```python
from build123d import *

# Parameters (mm, degrees)
F0_W     = 1004.8875
F0_H     = 609.6
F0_W_2   = 184.15
F0_H_2   = 95.25
F0_W_3   = 171.45
F0_H_3   = 88.9
F0_W_4   = 230.1875
F0_H_4   = 114.3
F0_H_5   = 60.325
F0_H_6   = 92.075
F1_DEPTH = 76.2
F2_W     = 1004.8875
F2_H     = 609.6
F3_DEPTH = 12.7
F5_DEPTH = 12.7


with BuildPart() as f1:
    # F0 (on Top) → F1 (new body)
    with BuildSketch(Plane.XY):
        with Locations((-595.931344, -92.764258)):
            Rectangle(F0_W, F0_H)
        with Locations((-993.600094, -337.239258)):
            Rectangle(F0_W_2, F0_H_2, mode=Mode.SUBTRACT)
        with Locations((-799.925094, -337.239258)):
            Rectangle(F0_W_2, F0_H_2, mode=Mode.SUBTRACT)
        with Locations((-612.600094, -340.414258)):
            Rectangle(F0_W_3, F0_H_3, mode=Mode.SUBTRACT)
        with Locations((-993.600094, -232.464258)):
            Rectangle(F0_W_2, F0_H_2, mode=Mode.SUBTRACT)
        with Locations((-993.600094, -127.689258)):
            Rectangle(F0_W_2, F0_H_2, mode=Mode.SUBTRACT)
        with Locations((-799.925094, -232.464258)):
            Rectangle(F0_W_2, F0_H_2, mode=Mode.SUBTRACT)
        with Locations((-612.600094, -241.989258)):
            Rectangle(F0_W_3, F0_H_3, mode=Mode.SUBTRACT)
        with Locations((-799.925094, -127.689258)):
            Rectangle(F0_W_2, F0_H_2, mode=Mode.SUBTRACT)
        with Locations((-612.600094, -143.564258)):
            Rectangle(F0_W_3, F0_H_3, mode=Mode.SUBTRACT)
        with Locations((-431.625094, -340.414258)):
            Rectangle(F0_W_3, F0_H_3, mode=Mode.SUBTRACT)
        with Locations((-221.281344, -327.714258)):
            Rectangle(F0_W_4, F0_H_4, mode=Mode.SUBTRACT)
        with Locations((-431.625094, -241.989258)):
            Rectangle(F0_W_3, F0_H_3, mode=Mode.SUBTRACT)
        with Locations((-431.625094, -143.564258)):
            Rectangle(F0_W_3, F0_H_3, mode=Mode.SUBTRACT)
        with Locations((-221.281344, -203.889258)):
            Rectangle(F0_W_4, F0_H_4, mode=Mode.SUBTRACT)
        with Locations((-993.600094, -22.914258)):
            Rectangle(F0_W_2, F0_H_2, mode=Mode.SUBTRACT)
        with Locations((-799.925094, -22.914258)):
            Rectangle(F0_W_2, F0_H_2, mode=Mode.SUBTRACT)
        with Locations((-612.600094, -45.139258)):
            Rectangle(F0_W_3, F0_H_3, mode=Mode.SUBTRACT)
        with Locations((-612.600094, 53.285742)):
            Rectangle(F0_W_3, F0_H_3, mode=Mode.SUBTRACT)
        with Locations((-993.600094, 81.860742)):
            Rectangle(F0_W_2, F0_H_2, mode=Mode.SUBTRACT)
        with Locations((-993.600094, 169.173242)):
            Rectangle(F0_W_2, F0_H_5, mode=Mode.SUBTRACT)
        with Locations((-799.925094, 81.860742)):
            Rectangle(F0_W_2, F0_H_2, mode=Mode.SUBTRACT)
        with Locations((-799.925094, 169.173242)):
            Rectangle(F0_W_2, F0_H_5, mode=Mode.SUBTRACT)
        with Locations((-612.600094, 153.298242)):
            Rectangle(F0_W_3, F0_H_6, mode=Mode.SUBTRACT)
        with Locations((-431.625094, -45.139258)):
            Rectangle(F0_W_3, F0_H_3, mode=Mode.SUBTRACT)
        with Locations((-431.625094, 53.285742)):
            Rectangle(F0_W_3, F0_H_3, mode=Mode.SUBTRACT)
        with Locations((-221.281344, -80.064258)):
            Rectangle(F0_W_4, F0_H_4, mode=Mode.SUBTRACT)
        with Locations((-221.281344, 43.760742)):
            Rectangle(F0_W_4, F0_H_4, mode=Mode.SUBTRACT)
        with Locations((-431.625094, 153.298242)):
            Rectangle(F0_W_3, F0_H_6, mode=Mode.SUBTRACT)
        with Locations((-221.281344, 154.885742)):
            Rectangle(F0_W_4, F0_H_3, mode=Mode.SUBTRACT)
    extrude(amount=F1_DEPTH)

    # F2 (on face) → F3 (join)
    with BuildSketch(Plane(origin=(0, 0, 0), x_dir=(1, 0, 0), z_dir=(0, 0, -1))):
        with Locations((-595.931344, 92.764258)):
            Rectangle(F2_W, F2_H)
    extrude(amount=F3_DEPTH)

    # F4 (on face) → F5 (join)
    with BuildSketch(Plane(origin=(0, 0, -12.7), x_dir=(1, 0, 0), z_dir=(0, 0, -1))):
        Polygon((-1098.375094, 397.564258), (-1098.375094, -212.035742), (-1085.675094, -212.035742), (-1085.675094, 384.864258), (-106.187594, 384.864258), (-106.187594, -212.035742), (-93.487594, -212.035742), (-93.487594, 397.564258), align=None)
    extrude(amount=F5_DEPTH)


solid = f1.part
```
Check sheet for the modelled part. Datum: model origin and axes. Units: mm. Give positions to 0.01 mm unless a question says otherwise; leave off trailing zeros. Write each loop counter-clockwise with the first axis right and the second up, starting at its lowest first coordinate (ties: lowest second). Pieces come first, ordered by that corner, then holes.
Item 1: Gauge pin test, flat ends, axial feed: pin 1 (6 mm diameter, centred on x = -897.5, y = -24.5, fed in from -Z); pin 2 (5 mm diameter, centred on x = -199, y = 24.5, fed in from +Z). Record the tip position at first contact, or that the pin passes through.
Item 2: Draft check along Y on faces 1 (the face through (-1085.675, -24, 38)), 2 (the face through (-1098.375, -97, 26)), 3 (the face through (-901.525, 169, 38)). Enter one of: released by +Y, released by -Y, zero draft, split by the parting line, or undercut.
Item 3: Scan lines: L1, parallel to X at y = -146.5, z = 4.5; L2, parallel to X at y = 36, z = 29.5; L3, parallel to Y at x = -320, z = 4. Record each from-to range of solid material in increasing order.
Item 4: Cross-section at A-A (x = -158.5). Enter the section's corners in (y, z).
Item 5: Cross-section at C-C (z = 60). Count the separate pieces of the cut face and the enclosed holes in it, and give its area (3 significant figures).
Item 6: Cross-section at B-B (y = -245). Enter the section's corners in (x, z), and give its area (3 significant figures).
Report:
1. pin 1: stops at z = -12.7
1. pin 2: stops at z = 0
2. face 1: undercut
2. face 2: zero draft
2. face 3: undercut
3. L1: x = -1098.38 to -1085.68, -901.53 to -892, -707.85 to -698.33, -526.88 to -517.35, -345.9 to -93.49
3. L2: x = -1098.38 to -1085.68, -901.53 to -892, -707.85 to -698.33, -526.88 to -517.35, -345.9 to -336.38, -106.19 to -93.49
3. L3: y = -397.56 to -384.86, -270.56 to -261.04, -146.74 to -137.21, -22.91 to -13.39, 100.91 to 110.44, 199.34 to 212.04
4. outline: (-397.56, -25.4) - (-384.86, -25.4) - (-384.86, -12.7) - (212.04, -12.7) - (212.04, 76.2) - (199.34, 76.2) - (199.34, 0) - (110.44, 0) - (110.44, 76.2) - (100.91, 76.2) - (100.91, 0) - (-13.39, 0) - (-13.39, 76.2) - (-22.91, 76.2) - (-22.91, 0) - (-137.21, 0) - (-137.21, 76.2) - (-146.74, 76.2) - (-146.74, 0) - (-261.04, 0) - (-261.04, 76.2) - (-270.56, 76.2) - (-270.56, 0) - (-384.86, 0) - (-384.86, 76.2) - (-397.56, 76.2) - close
5. separate pieces: 1
5. enclosed holes: 29
5. area: 105,000 mm2
6. outline: (-1098.38, -25.4) - (-1085.68, -25.4) - (-1085.68, -12.7) - (-106.19, -12.7) - (-106.19, -25.4) - (-93.49, -25.4) - (-93.49, 76.2) - (-106.19, 76.2) - (-106.19, 0) - (-336.38, 0) - (-336.38, 76.2) - (-345.9, 76.2) - (-345.9, 0) - (-517.35, 0) - (-517.35, 76.2) - (-526.88, 76.2) - (-526.88, 0) - (-698.33, 0) - (-698.33, 76.2) - (-707.85, 76.2) - (-707.85, 0) - (-892, 0) - (-892, 76.2) - (-901.53, 76.2) - (-901.53, 0) - (-1085.68, 0) - (-1085.68, 76.2) - (-1098.38, 76.2) - close
6. area: 17,900 mm2
